Check sheet for the modelled part. Datum: model origin and axes. Units: mm. A direction names the side the tool comes from. Give positions to 0.01 mm unless a question says otherwise; leave off trailing zeros. Order: outer loops, then holes, each group sorted by start corner. A loop starts at its lowest first (then second) coordinate and runs counter-clockwise, first axis right, second up.
from build123d import *

# Parameters (mm, degrees)
SKETCH1_W                                         = 57.15
SKETCH1_H                                         = 57.15
BOSS_EXTRUDE2_DEPTH                               = 6.35
FILLET1_R                                         = 5.08
SKETCH2_R                                         = 19.05
CUT_EXTRUDE1_DEPTH                                = 1.524
CSK_FOR_1_FLAT_HEAD_MACHINE_SCREW_100_D           = 5.08
CSK_FOR_1_FLAT_HEAD_MACHINE_SCREW_100_CSINK_D     = 7.62
CSK_FOR_1_FLAT_HEAD_MACHINE_SCREW_100_CSINK_ANGLE = 90
SKETCH14_R                                        = 3.175
CUT_EXTRUDE2_DEPTH                                = 4.826
FILLET2_R                                         = 1.016
SKETCH15_R                                        = 16.764
CUT_EXTRUDE4_DEPTH                                = 4.826


with BuildPart() as part:
    # Sketch1 → Boss-Extrude2 (new body)
    with BuildSketch(Plane(origin=(0, 0, 0), x_dir=(1, 0, 0), z_dir=(0, 1, 0))):
        Rectangle(SKETCH1_W, SKETCH1_H)
    extrude(amount=BOSS_EXTRUDE2_DEPTH)

    # Fillet1
    fillet1_edges = [part.edges().sort_by_distance(p)[0] for p in [
        (28.575, 3.175, 28.575),
        (-28.575, 3.175, 28.575),
        (-28.575, 3.175, -28.575),
        (28.575, 3.175, -28.575),
    ]]
    fillet(fillet1_edges, radius=FILLET1_R)

    # Sketch2 → Cut-Extrude1 (cut)
    with BuildSketch(Plane.XZ):
        with Locations(Location((0, 0, 0), (0, 0, 270))):
            Circle(SKETCH2_R)
    extrude(amount=-CUT_EXTRUDE1_DEPTH, mode=Mode.SUBTRACT)

    # CSK for #1 Flat Head Machine Screw (100)2 (through all)
    with Locations(Plane(origin=(0, 6.35, 0), x_dir=(1, 0, 0), z_dir=(0, 1, 0))):
        with Locations((-23.495, 23.495), (23.495, 23.495), (-23.495, -23.495), (23.495, -23.495)):
            CounterSinkHole(CSK_FOR_1_FLAT_HEAD_MACHINE_SCREW_100_D / 2, CSK_FOR_1_FLAT_HEAD_MACHINE_SCREW_100_CSINK_D / 2, counter_sink_angle=CSK_FOR_1_FLAT_HEAD_MACHINE_SCREW_100_CSINK_ANGLE)

    # Sketch14 → Cut-Extrude2 (cut)
    with BuildSketch(Plane(origin=(0, 6.35, 0), x_dir=(1, 0, 0), z_dir=(0, 1, 0))):
        with Locations(Location((0, 0, 0), (0, 0, 270))):
            Circle(SKETCH14_R)
    extrude(amount=-CUT_EXTRUDE2_DEPTH, mode=Mode.SUBTRACT)

    # Fillet2
    fillet2_edges = [part.edges().sort_by_distance(p)[0] for p in [
        (0, 6.35, 28.575),
        (-28.575, 6.35, 0),
        (28.575, 6.35, 0),
        (0, 6.35, -28.575),
        (-27.087102448, 6.35, -27.087102448),
        (27.087102448, 6.35, -27.087102448),
        (27.087102448, 6.35, 27.087102448),
        (-27.087102448, 6.35, 27.087102448),
    ]]
    fillet(fillet2_edges, radius=FILLET2_R)

    # Sketch15 → Cut-Extrude4 (cut)
    with BuildSketch(Plane(origin=(0, 6.35, 0), x_dir=(1, 0, 0), z_dir=(0, 1, 0))):
        with Locations(Location((0, 0, 0), (0, 0, 270))):
            Circle(SKETCH15_R)
    extrude(amount=-CUT_EXTRUDE4_DEPTH, mode=Mode.SUBTRACT)


solid = part.part
1) Section check A-A, the plane z = 0. Record the cut outline in (x, y) (3 decimals), then the cut area to 3 significant figures.
Recorded:
outline: (-28.575, 0) - (-19.05, 0) - (-19.05, 1.524) - (-16.764, 1.524) - (-16.764, 6.35) - (-27.559, 6.35) arc R1.016 ccw to (-28.575, 5.334) - close; (16.764, 1.524) - (19.05, 1.524) - (19.05, 0) - (28.575, 0) - (28.575, 5.334) arc R1.016 ccw to (27.559, 6.35) - (16.764, 6.35) - close
area: 143 mm2
2) Material ranges on L1, parallel to X at y = 5, z = 23.5 (3 decimals); L2, parallel to X at y = 0.4, z = 0 (3 decimals); L3, parallel to X at y = 1.75, z = -25, recorded low to high.
Recorded:
L1: x = -28.575 to -26.035, -20.955 to 20.955, 26.035 to 28.575
L2: x = -28.575 to -19.05, 19.05 to 28.575
L3: x = -28.35 to -25.54, -21.45 to 21.45, 25.54 to 28.35
3) Section check B-B, the plane y = 2.5. Record the cut outline in (x, z) (3 decimals).
Recorded:
outline: (-28.575, -23.495) arc R5.08 ccw to (-23.495, -28.575) - (23.495, -28.575) arc R5.08 ccw to (28.575, -23.495) - (28.575, 23.495) arc R5.08 ccw to (23.495, 28.575) - (-23.495, 28.575) arc R5.08 ccw to (-28.575, 23.495) - close; hole circle Ø5.08 at (-23.495, -23.495); hole circle Ø5.08 at (-23.495, 23.495); hole circle Ø33.528 at (0, 0); hole circle Ø5.08 at (23.495, -23.495); hole circle Ø5.08 at (23.495, 23.495)
4) Section check C-C, the plane x = 0. Record the cut outline in (y, z) (3 decimals), then the cut area to 3 significant figures.
Recorded:
outline: (0, -28.575) - (5.334, -28.575) arc R1.016 ccw to (6.35, -27.559) - (6.35, -16.764) - (1.524, -16.764) - (1.524, -19.05) - (0, -19.05) - close; (0, 19.05) - (1.524, 19.05) - (1.524, 16.764) - (6.35, 16.764) - (6.35, 27.559) arc R1.016 ccw to (5.334, 28.575) - (0, 28.575) - close
area: 143 mm2
5) Set-up check for faces 1 (the face through (0, 3, 28.575)), 2 (the face through (-11.59, 0.75, 15.12)): record each of +Z, -Z, +X, -X, +Y, -Y from which the full face is reachable in a straight line by a thin tool's end or side.
Recorded:
face 1: +Z, +X, -X, +Y, -Y
face 2: -Y
6) Depth check by flat-ended pin: pin 1 Ø8 at (x, z) = (-23.495, 23.495) entering from -Y. Enter the tip coordinate at first touch or a pass-through.
Recorded:
pin 1: stops at y = 0
7) Draft check along X on faces 3 (the face through (24.046, 2.504, -21.015)), 4 (the face through (28.575, 3, 0)), 5 (the face through (-10.201, 3.971, -13.303)), 6 (the face through (0, 3, -28.575)). Enter one of: +X half, -X half, draft (parallel to the pull), parting line (faces both ways), or undercut.
Recorded:
face 3: undercut
face 4: +X half
face 5: undercut
face 6: draft
